```python
from build123d import *

# Parameters (mm, degrees)
F1_W = 1.5
F1_H = 19.0184637904


with BuildPart() as f2:
    # F1 (on Right) → F2 (revolve)
    with BuildSketch(Plane.YZ):
        Polygon((-14.2185513526, 19.0184637904), (-14.2185513526, 24.0184637904), (-15.7185513526, 24.0184637904), (-17.4685513526, 24.0184637904), (-15.7185513526, 19.0184637904), align=None)
        Polygon((-15.7185513526, 24.0184637904), (-14.2185513526, 24.0184637904), (-7.4561595252, 100.0857525279), (-8.9502772316, 100.2184637904), align=None)
        with Locations((-14.9685513526, 9.5092318952)):
            Rectangle(F1_W, F1_H)
    revolve(axis=Axis((0, 0, 0), (0, 0, 1)))


solid = f2.part
```
Can you work these out from the model? Positions are in its coordinate system, mm. A direction names the side the tool comes from. Give positions to 0.01 mm unless a question says otherwise; leave off trailing zeros. Loops run counter-clockwise (first coordinate to the right, second up) from the corner with the lowest first, then second, coordinate; pieces in that order, holes last. Notation, with made-up numbers: M 6.25,58 L 33.25,58 A27 ccw 33.25,93 Z; hole C 38,-12 d11. An arc over 180 degrees is marked long. One line per item, written item: value.
(1) Suppose I cut it at A-A on y = 0. List the corners of the cut face in (x, z) for me.
Returned:
outline: M -17.47,24.02 L -15.72,19.02 L -15.72,0 L -14.22,0 L -14.22,24.02 L -7.46,100.09 L -8.95,100.22 L -15.72,24.02 Z; M 7.46,100.09 L 14.22,24.02 L 14.22,0 L 15.72,0 L 15.72,19.02 L 17.47,24.02 L 15.72,24.02 L 8.95,100.22 Z
(2) Will these pins go through, and if not, where does the flat tip stop? pin 1 (8 mm diameter, centred on x = 11.5, z = 15.5, fed in from -Y); pin 2 (2 mm diameter, centred on x = -12.5, z = 46.5, fed in from +Y); pin 3 (10 mm diameter, centred on y = -7, z = 52, fed in from -X).
Returned:
pin 1: y = -13.81
pin 2: y = 7.49
pin 3: x = -13.19
(3) Suppose I cut it at D-D on z = 63. List the corners of the cut face in (x, y) for me, plus the area to 3 significant figures.
Returned:
outline: C 0,0 d24.51; hole C 0,0 d21.51
area: 109 mm^2
(4) Suppose I cut it at C-C on z = 10. List the corners of the cut face in (x, y) for me.
Returned:
outline: C 0,0 d31.44; hole C 0,0 d28.44
(5) Which directions (+Z, -Z, +X, -X, +Y, -Y) give clear straight access to the entire face, cutting with the end or side of a thin tool? Please do faces 4 (the face through (11.99, -7.64, 12.18)), 5 (the face through (3, -16, 24.018)).
Returned:
face 4: -Z
face 5: +Z
(6) We'd pull the mould along Y, two halves only. Please class faces 1 (the face through (-6.57, 8.56, 62.58)), 2 (the face through (-15.345, 3.407, 9.642)), 3 (the face through (-8, 12, 0)): released by +Y, released by -Y, zero draft, split by the parting line, or undercut.
Returned:
face 1: undercut
face 2: split by the parting line
face 3: zero draft
(7) I need wall thicknesses on line 1 (X direction, y = 0, z = 5); line 2 (Y direction, x = 4.5, z = 14); line 3 (X direction, y = 7, z = 25.5). Which ranges of each line are inside material? Lowest first, please.
Returned:
line 1: -15.72 to -14.22, 14.22 to 15.72
line 2: -15.06 to -13.49, 13.49 to 15.06
line 3: -13.93 to -12.22, 12.22 to 13.93
